For this review, take the finished solid that the model builds, in its own axes (mm). A direction names the side the tool comes from. Coordinates: 2 decimals unless noted, no trailing zeros. Write each loop counter-clockwise with the first axis right and the second up, starting at its lowest first coordinate (ties: lowest second). Pieces come first, ordered by that corner, then holes. Notation, with made-up numbers: M 80,49.25 L 131,49.25 A24 ccw 131,88.25 Z; hole C 65.5,82.25 d2. An arc over 180 degrees is marked long. Return JSON: item names as keys, results as strings.
Autodesk Inventor part; units mm, degrees
ref_plane "YZ Plane" through (0, 0, 0) normal (1, 0, 0) x (0, 1, 0)
ref_plane "XZ Plane" through (0, 0, 0) normal (0, 1, 0) x (-1, 0, 0)
ref_plane "XY Plane" through (0, 0, 0) normal (0, 0, 1) x (1, 0, 0)
sketch "Skizze1" plane through (0, 0, 0) normal (0, 0, 1) x (1, 0, 0)
  line L0 (-21, 0) -> (21, 0)
  line L1 (0, -21) -> (0, 21)
  circle A0 centre (0, 0) radius 15
  dimension "d0" = 30
extrude "Extrusion1" add sketch "Skizze1" along normal blind 40
sketch "Skizze2" plane through (0, 0, 40) normal (0, 0, 1) x (1, 0, 0)
  circle A0 centre (0, 0) radius 10
  dimension "d3" = 20
extrude "Extrusion2" add sketch "Skizze2" along normal blind 40
thread "Gewinde1"
thread "Gewinde2"
chamfer "Fase1" distance 0.5 angle 45 1 edges at (-15, 0, 40)
sketch "Skizze3" plane through (0, 0, 80) normal (0, 0, 1) x (1, 0, 0)
  circle A0 centre (0, 0) radius 9
  dimension "d13" = 18
extrude "Extrusion3" cut sketch "Skizze3" against normal blind 80
chamfer "Fase2" distance 0.5 angle 45 3 edges at (-10, 0, 80) (-9, 0, 0) (-15, 0, 0)
properties part number "Durchflusssensor"
1. Wall thickness on L1, parallel to Y at x = 0, z = 17; L2, parallel to X at y = 3, z = 9; L3, parallel to X at y = 3, z = 67.5: over which ranges is each line inside the solid? List them lowest first. Write a range as from..to.
Checks:
{"L1": "-15..-9, 9..15", "L2": "-14.7..-8.49, 8.49..14.7", "L3": "-9.54..-8.49, 8.49..9.54"}
2. We need section A-A (y = 0). State the section outline as (x, z) points, plus the area to 3 significant figures.
Checks:
{"outline": "M -15,0.5 L -14.5,0 L -9.5,0 L -9,0.5 L -9,80 L -9.5,80 L -10,79.5 L -10,40 L -14.5,40 L -15,39.5 Z; M 9,0.5 L 9.5,0 L 14.5,0 L 15,0.5 L 15,39.5 L 14.5,40 L 10,40 L 10,79.5 L 9.5,80 L 9,80 Z", "area": "559 mm2"}
3. For faces 1 (the face through (-14.985, -0.66, 19.727)), 2 (the face through (3, 10, 40)), list the 3-axis set-ups (+Z, -Z, +X, -X, +Y, -Y) from which the entire face can be reached by the end or side of a thin tool; tool diameter is ignored.
Checks:
{"face 1": "+Z, -Z", "face 2": "+Z"}
4. Clearance check with flat-ended pins moving along their axes: pin 1 Ø4 at (y, z) = (1.5, 43.5) entering from -X; pin 2 Ø10 at (y, z) = (-11, 34.5) entering from -X; pin 3 Ø1 at (y, z) = (7, 25.5) entering from +X. State where each tip first meets the part, or that it passes through.
Checks:
{"pin 1": "x = -10", "pin 2": "x = -13.75", "pin 3": "x = 13.52"}
5. We need section C-C (z = 13.5). State the section outline as (x, y) points, plus the area to 3 significant figures.
Checks:
{"outline": "C 0,0 d30; hole C 0,0 d18", "area": "452 mm2"}
6. Draft analysis for pull direction Y (two halves, no side actions). For faces 3 (the face through (-6, -7, 80)), 4 (the face through (-1.172, 8.923, 40.806)), 5 (the face through (-2.17, 9.76, 59.47)), state which applies: +Y half, -Y half, draft (parallel to the pull), parting line (faces both ways), or undercut.
Checks:
{"face 3": "draft", "face 4": "undercut", "face 5": "parting line"}
